from build123d import *

# Parameters (mm, degrees)
SKETCH1_W           = 61.0616
SKETCH1_H           = 40.64
BOSS_EXTRUDE1_DEPTH = 82.55
SKETCH13_W          = 54.7116
SKETCH13_H          = 34.29
CUT_EXTRUDE1_DEPTH  = 82.55
SKETCH15_R          = 14.478
CUT_EXTRUDE2_DEPTH  = 3.175
CUT_EXTRUDE3_START  = -37.465
SKETCH16_R          = 14.478
CUT_EXTRUDE3_DEPTH  = 3.175
CUT_EXTRUDE4_START  = -61.0616
SKETCH18_R          = 14.478
CUT_EXTRUDE4_DEPTH  = 61.0616
CUT_EXTRUDE5_START  = -40.64
SKETCH19_W          = 19.05
SKETCH19_H          = 34.925
CUT_EXTRUDE5_DEPTH  = 40.64
CUT_EXTRUDE6_START  = -40.64
SKETCH20_R          = 2.413
CUT_EXTRUDE6_DEPTH  = 40.64
CUT_EXTRUDE7_START  = -40.64
SKETCH21_R          = 2.413
CUT_EXTRUDE7_DEPTH  = 40.64
CUT_EXTRUDE8_START  = -40.64
SKETCH24_R          = 2.413
CUT_EXTRUDE8_DEPTH  = 40.64
CUT_EXTRUDE9_START  = -40.64
SKETCH25_R          = 2.413
CUT_EXTRUDE9_DEPTH  = 40.64
BOSS_EXTRUDE2_DEPTH = 6.35
BOSS_EXTRUDE3_DEPTH = 6.35
SKETCH53_W          = 61.0616
SKETCH53_H          = 40.64
SKETCH53_W_2        = 54.7116
SKETCH53_H_2        = 34.29
BOSS_EXTRUDE5_DEPTH = 3.175
SKETCH54_W          = 61.0616
SKETCH54_H          = 40.64
BOSS_EXTRUDE6_DEPTH = 3.175
CUT_EXTRUDE14_START = -40.64
SKETCH45_R          = 2.413
CUT_EXTRUDE14_DEPTH = 40.64
CUT_EXTRUDE18_START = -40.64
SKETCH59_R          = 2.413
CUT_EXTRUDE18_DEPTH = 40.64
CUT_EXTRUDE19_START = -40.64
SKETCH60_R          = 2.413
CUT_EXTRUDE19_DEPTH = 40.64
CUT_EXTRUDE20_START = -40.64
SKETCH61_R          = 2.413
CUT_EXTRUDE20_DEPTH = 40.64
CUT_EXTRUDE21_START = -61.0616
SKETCH63_R          = 2.413
CUT_EXTRUDE21_DEPTH = 61.0616
CUT_EXTRUDE22_START = -61.0616
SKETCH64_R          = 2.413
CUT_EXTRUDE22_DEPTH = 61.0616
CUT_EXTRUDE23_START = -61.0616
SKETCH65_R          = 2.413
CUT_EXTRUDE23_DEPTH = 61.0616
CUT_EXTRUDE24_START = -61.0616
SKETCH66_R          = 2.413
CUT_EXTRUDE24_DEPTH = 61.0616


with BuildPart() as part:
    # Sketch1 → Boss-Extrude1 (new body)
    with BuildSketch(Plane(origin=(0, 0, 0), x_dir=(1, 0, 0), z_dir=(0, 1, 0))):
        with Locations((30.5308, 20.32)):
            Rectangle(SKETCH1_W, SKETCH1_H)
    extrude(amount=BOSS_EXTRUDE1_DEPTH)

    # Sketch13 → Cut-Extrude1 (cut)
    with BuildSketch(Plane(origin=(0, 82.55, 0), x_dir=(1, 0, 0), z_dir=(0, 1, 0))):
        with Locations((30.5308, 20.32)):
            Rectangle(SKETCH13_W, SKETCH13_H)
    extrude(amount=-CUT_EXTRUDE1_DEPTH, mode=Mode.SUBTRACT)

    # Sketch15 → Cut-Extrude2 (cut)
    with BuildSketch(Plane.XY):
        with Locations((30.5308, 31.75)):
            Circle(SKETCH15_R)
    extrude(amount=-CUT_EXTRUDE2_DEPTH, mode=Mode.SUBTRACT)

    # Sketch16 → Cut-Extrude3 (cut)
    with BuildSketch(Plane.XY.offset(CUT_EXTRUDE3_START)):
        with Locations((30.5308, 31.75)):
            Circle(SKETCH16_R)
    extrude(amount=-CUT_EXTRUDE3_DEPTH, mode=Mode.SUBTRACT)

    # Sketch18 → Cut-Extrude4 (cut)
    with BuildSketch(Plane.ZY.offset(CUT_EXTRUDE4_START)):
        with Locations((-20.32, 63.754)):
            Circle(SKETCH18_R)
    extrude(amount=CUT_EXTRUDE4_DEPTH, mode=Mode.SUBTRACT)

    # Sketch19 → Cut-Extrude5 (cut)
    with BuildSketch(Plane(origin=(0, 0, -40.64), x_dir=(-1, 0, 0), z_dir=(0, 0, -1)).offset(CUT_EXTRUDE5_START)):
        with Locations((-30.5308, 65.0875)):
            Rectangle(SKETCH19_W, SKETCH19_H)
    extrude(amount=CUT_EXTRUDE5_DEPTH, mode=Mode.SUBTRACT)

    # Sketch20 → Cut-Extrude6 (cut)
    with BuildSketch(Plane.XY.offset(CUT_EXTRUDE6_START)):
        with Locations((48.26, 14.0208)):
            Circle(SKETCH20_R)
    extrude(amount=CUT_EXTRUDE6_DEPTH, mode=Mode.SUBTRACT)

    # Sketch21 → Cut-Extrude7 (cut)
    with BuildSketch(Plane.XY.offset(CUT_EXTRUDE7_START)):
        with Locations((48.26, 49.473689268)):
            Circle(SKETCH21_R)
    extrude(amount=CUT_EXTRUDE7_DEPTH, mode=Mode.SUBTRACT)

    # Sketch24 → Cut-Extrude8 (cut)
    with BuildSketch(Plane.XY.offset(CUT_EXTRUDE8_START)):
        with Locations((12.807110732, 49.473689268)):
            Circle(SKETCH24_R)
    extrude(amount=CUT_EXTRUDE8_DEPTH, mode=Mode.SUBTRACT)

    # Sketch25 → Cut-Extrude9 (cut)
    with BuildSketch(Plane.XY.offset(CUT_EXTRUDE9_START)):
        with Locations((12.807110732, 14.0208)):
            Circle(SKETCH25_R)
    extrude(amount=CUT_EXTRUDE9_DEPTH, mode=Mode.SUBTRACT)

    # Sketch47 → Boss-Extrude2 (add)
    with BuildSketch(Plane(origin=(0, 82.55, 0), x_dir=(1, 0, 0), z_dir=(0, 1, 0))):
        Polygon((21.0058, 40.64), (21.0058, 37.465), (3.175, 37.465), (3.175, 3.175), (21.0058, 3.175), (21.0058, 0), (0, 0), (0, 40.64), (20.248497821, 40.64), align=None)
    extrude(amount=BOSS_EXTRUDE2_DEPTH)

    # Sketch49 → Boss-Extrude3 (add)
    with BuildSketch(Plane(origin=(0, 82.55, 0), x_dir=(1, 0, 0), z_dir=(0, 1, 0))):
        Polygon((40.0558, 37.465), (40.0558, 40.64), (61.0616, 40.64), (61.0616, 0), (40.224521991, 0), (40.0558, 3.175), (57.8866, 3.175), (57.8866, 37.465), align=None)
    extrude(amount=BOSS_EXTRUDE3_DEPTH)

    # Sketch53 → Boss-Extrude5 (add)
    with BuildSketch(Plane.XZ):
        with Locations((30.5308, -20.32)):
            Rectangle(SKETCH53_W, SKETCH53_H)
        with Locations((30.5308, -20.32)):
            Rectangle(SKETCH53_W_2, SKETCH53_H_2, mode=Mode.SUBTRACT)
    extrude(amount=BOSS_EXTRUDE5_DEPTH)

    # Sketch54 → Boss-Extrude6 (add)
    with BuildSketch(Plane.XZ.offset(3.175)):
        with Locations((30.5308, -20.32)):
            Rectangle(SKETCH54_W, SKETCH54_H)
    extrude(amount=BOSS_EXTRUDE6_DEPTH)

    # Sketch45 → Cut-Extrude14 (cut)
    with BuildSketch(Plane.XY.offset(CUT_EXTRUDE14_START)):
        with Locations((49.5808, 6.35)):
            Circle(SKETCH45_R)
    extrude(amount=CUT_EXTRUDE14_DEPTH, mode=Mode.SUBTRACT)

    # Sketch59 → Cut-Extrude18 (cut)
    with BuildSketch(Plane.XY.offset(CUT_EXTRUDE18_START)):
        with Locations((49.5808, 82.55)):
            Circle(SKETCH59_R)
    extrude(amount=CUT_EXTRUDE18_DEPTH, mode=Mode.SUBTRACT)

    # Sketch60 → Cut-Extrude19 (cut)
    with BuildSketch(Plane.XY.offset(CUT_EXTRUDE19_START)):
        with Locations((11.4808, 6.35)):
            Circle(SKETCH60_R)
    extrude(amount=CUT_EXTRUDE19_DEPTH, mode=Mode.SUBTRACT)

    # Sketch61 → Cut-Extrude20 (cut)
    with BuildSketch(Plane.XY.offset(CUT_EXTRUDE20_START)):
        with Locations((11.4808, 82.55)):
            Circle(SKETCH61_R)
    extrude(amount=CUT_EXTRUDE20_DEPTH, mode=Mode.SUBTRACT)

    # Sketch63 → Cut-Extrude21 (cut)
    with BuildSketch(Plane.ZY.offset(CUT_EXTRUDE21_START)):
        with Locations((-33.02, 82.55)):
            Circle(SKETCH63_R)
    extrude(amount=CUT_EXTRUDE21_DEPTH, mode=Mode.SUBTRACT)

    # Sketch64 → Cut-Extrude22 (cut)
    with BuildSketch(Plane.ZY.offset(CUT_EXTRUDE22_START)):
        with Locations((-7.62, 82.55)):
            Circle(SKETCH64_R)
    extrude(amount=CUT_EXTRUDE22_DEPTH, mode=Mode.SUBTRACT)

    # Sketch65 → Cut-Extrude23 (cut)
    with BuildSketch(Plane.ZY.offset(CUT_EXTRUDE23_START)):
        with Locations((-30.607, 6.35)):
            Circle(SKETCH65_R)
    extrude(amount=CUT_EXTRUDE23_DEPTH, mode=Mode.SUBTRACT)

    # Sketch66 → Cut-Extrude24 (cut)
    with BuildSketch(Plane.ZY.offset(CUT_EXTRUDE24_START)):
        with Locations((-7.62, 6.35)):
            Circle(SKETCH66_R)
    extrude(amount=CUT_EXTRUDE24_DEPTH, mode=Mode.SUBTRACT)


solid = part.part
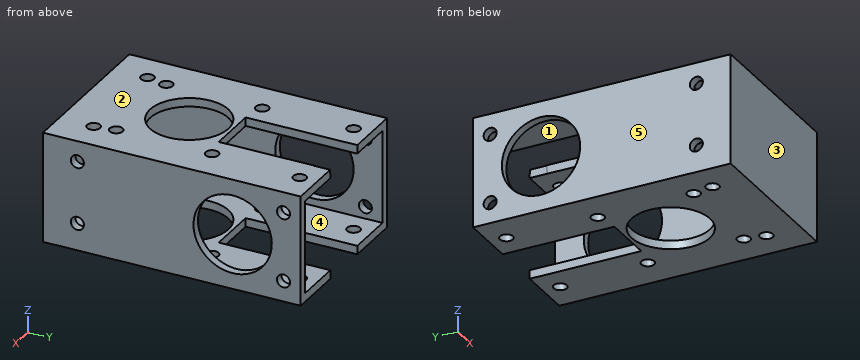
Geometry: final body of the model. Coordinates: model frame, mm. Face numbers are marked on the shaded views. A direction names the side the tool comes from. Coordinates: 2 decimals unless noted, no trailing zeros. Order: outer loops, then holes, each group sorted by start corner. A loop starts at its lowest first (then second) coordinate and runs counter-clockwise, first axis right, second up. Notation, with made-up numbers: M -2,66.5 L 10,66.5 A29 cw 10,99.5 Z; hole C 64.25,78.25 d4. An arc over 180 degrees is marked long. One line per question, with ' | ' between items. Start each with the question number.
Item 1: Draft query along Z for the marked faces 1, 2 and 3. Return one class per face: released by +Z, released by -Z, zero draft, split by the parting line, or undercut.
Item 2: Pin query (flat end, axial travel): pin 1 Ø3 at (y, z) = (6.35, -30.607) entering from +X; pin 2 Ø1 at (x, z) = (54.5, -7) entering from +Y (3 decimals); pin 3 Ø3.5 at (x, z) = (34.5, -39) entering from +Y (3 decimals). Return the tip coordinate at first contact, or that it passes through.
Item 3: Cut plane D-D, the plane y = 55.5. Return the cut outline in (x, z) (3 decimals).
Item 4: Cut plane C-C, the plane x = 26. Return the cut outline in (y, z) (3 decimals).
Item 5: Ray query, probe 1 along Z at (x, y) = (60, 82.55); probe 2 along Z at (x, y) = (55, 27) (3 decimals); probe 3 along X at (y, z) = (81, -12) (3 decimals). Return the intervals inside material, ascending. Write a range as [from, to].
Item 6: Set-up query: the marked faces 4 and 5. Return all of +Z, -Z, +X, -X, +Y, -Y with unobstructed straight access to the full face (end or side cutting, diameter ignored); none if empty.
Item 7: Cut plane B-B, the plane y = 10. Return the cut outline in (x, z) (3 decimals).
Item 8: Cut plane A-A, the plane z = -20.32. Return the cut outline in (x, y) (3 decimals).
A:
1) face 1: undercut | face 2: released by +Z | face 3: zero draft
2) pin 1: passes through | pin 2: stops at y = -3.175 | pin 3: stops at y = 47.625
3) outline: M 0,-40.64 L 21.006,-40.64 L 21.006,-37.465 L 3.175,-37.465 L 3.175,-32.215 L 0,-32.215 Z; M 0,-8.425 L 3.175,-8.425 L 3.175,-3.175 L 21.006,-3.175 L 21.006,0 L 0,0 Z; M 40.056,-40.64 L 61.062,-40.64 L 61.062,-32.215 L 57.887,-32.215 L 57.887,-37.465 L 40.056,-37.465 Z; M 40.056,-3.175 L 57.887,-3.175 L 57.887,-8.425 L 61.062,-8.425 L 61.062,0 L 40.056,0 Z
4) outline: M -6.35,-40.64 L 17.999,-40.64 L 17.999,-37.465 L -3.175,-37.465 L -3.175,-3.175 L 17.999,-3.175 L 17.999,0 L -6.35,0 Z; M 45.501,-40.64 L 47.625,-40.64 L 47.625,-37.465 L 45.501,-37.465 Z; M 45.501,-3.175 L 47.625,-3.175 L 47.625,0 L 45.501,0 Z
5) probe 1: z = [-40.64, -35.43], [-30.61, -10.03], [-5.21, 0] | probe 2: z = [-40.64, -37.465], [-3.175, 0] | probe 3: x = [0, 3.175], [57.887, 61.062]
6) face 4: +Y | face 5: +Z, -Z, -X, +Y, -Y
7) outline: M 0,-40.64 L 61.062,-40.64 L 61.062,0 L 0,0 Z; hole M 3.175,-37.465 L 57.887,-37.465 L 57.887,-3.175 L 3.175,-3.175 Z
8) outline: M 0,-6.35 L 61.062,-6.35 L 61.062,49.276 L 57.887,49.276 L 57.887,-3.175 L 3.175,-3.175 L 3.175,49.276 L 0,49.276 Z; M 0,78.232 L 3.175,78.232 L 3.175,88.9 L 0,88.9 Z; M 57.887,78.232 L 61.062,78.232 L 61.062,88.9 L 57.887,88.9 Z
